Input: part model. Units: mm. Frame: model coordinates. Coordinates: 2 decimals unless noted, no trailing zeros. Write each loop counter-clockwise with the first axis right and the second up, starting at its lowest first coordinate (ties: lowest second). Pieces come first, ordered by that corner, then holes. Notation, with made-up numbers: (-23.75, 23.5) - (7.25, 23.5) arc R30 ccw to (7.25, 57.5) - close; hole circle Ø9 at (3, 20). An arc over 180 degrees is marked (long way). Use a Markdown table: item, result. Add a question column.
Q1. Material intervals for probe 1 along Z at (x, y) = (46, 61); probe 2 along X at (y, z) = (218.5, 7.25); probe 3 along Y at (x, z) = (10, 12), sorted ascending. Write a range as from..to.
Q2. Section query B-B (x = 13). Return the cut outline in (y, z), then the cut area to 3 significant figures.
Q3. Section query A-A (y = 56). Return the cut outline in (x, z).
Q4. Pin query (flat end, axial travel): P1, Ø5, axis at y = 260, z = 9.5, coming from the +X side; P2, Ø5, axis at x = 13, z = 12, coming from the -Y side; P3, Ø3, axis at x = 32, z = 11, coming from the -Y side. Return the tip coordinate at first contact, or that it passes through.
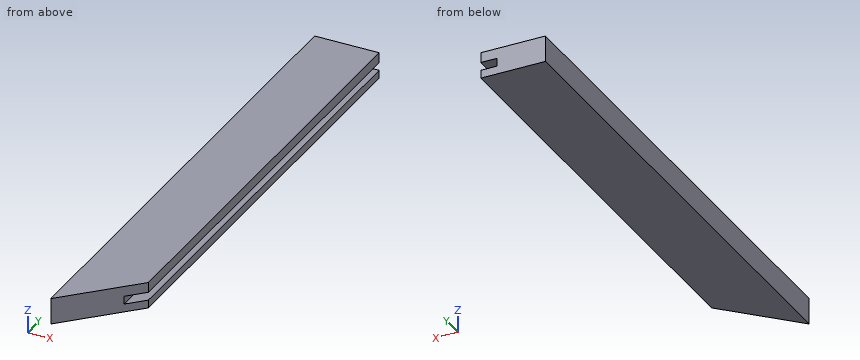
from build123d import *

# Parameters (mm, degrees)
F1_DEPTH = 20.6375
F2_W     = 12.7
F2_H     = 6.35
F3_DEPTH = 406.401


with BuildPart() as f1:
    # F0 (on Top) → F1 (new body)
    with BuildSketch(Plane.XY):
        Polygon((50.8, 406.4), (0, 406.4), (0, 0), (50.8, 50.8), align=None)
    extrude(amount=F1_DEPTH)

    # F2 (on face) → F3 (cut, through all)
    with BuildSketch(Plane(origin=(0, 406.4, 0), x_dir=(-1, 0, 0), z_dir=(0, 1, 0))):
        with Locations((-44.45, 9.525)):
            Rectangle(F2_W, F2_H)
    extrude(amount=-F3_DEPTH, mode=Mode.SUBTRACT)


solid = f1.part
Values follow:
| question | item | result |
|---|---|---|
| 1 | probe 1 | 0..6.35, 12.7..20.64 |
| 1 | probe 2 | 0..38.1 |
| 1 | probe 3 | 10..406.4 |
| 2 | outline | (13, 0) - (406.4, 0) - (406.4, 20.64) - (13, 20.64) - close |
| 2 | area | 8,120 mm2 |
| 3 | outline | (0, 0) - (50.8, 0) - (50.8, 6.35) - (38.1, 6.35) - (38.1, 12.7) - (50.8, 12.7) - (50.8, 20.64) - (0, 20.64) - close |
| 4 | P1 | x = 38.1 |
| 4 | P2 | y = 10.5 |
| 4 | P3 | y = 30.5 |
